Can you work these out from the model? Positions are in its coordinate system, mm. Face numbers are marked on the shaded views. A direction names the side the tool comes from. Give positions to 0.01 mm unless a question says otherwise; leave off trailing zeros. Write each loop counter-clockwise with the first axis right and the second up, starting at its lowest first coordinate (ties: lowest second). Pieces come first, ordered by that corner, then holes. Notation, with made-up numbers: (61, 8) -> (93, 8) arc R29 ccw to (93, 38) -> close; hole circle Ø4 at (16.5, 6.5). An arc over 180 degrees is marked (long way). One line per item, written item: value.
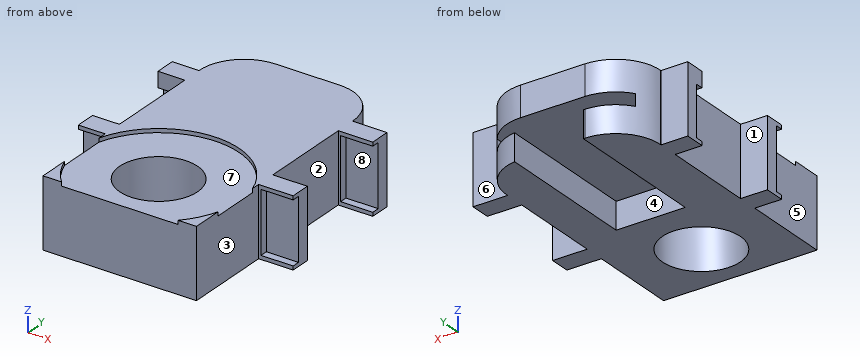
from build123d import *

# Parameters (mm, degrees)
SKETCH2_W           = 20
SKETCH2_H           = 35
BOSS_EXTRUDE1_DEPTH = 9
SKETCH3_W           = 9
SKETCH3_H           = 2.65
BOSS_EXTRUDE2_DEPTH = 14
SKETCH3_2_W         = 9
SKETCH3_2_H         = 2.65
BOSS_EXTRUDE3_DEPTH = 14
SKETCH4_R           = 5.075
CUT_EXTRUDE1_DEPTH  = 10
SKETCH5_R           = 10.5
CUT_EXTRUDE2_DEPTH  = 0.5
SKETCH7_W           = 18
SKETCH7_H           = 1.55
CUT_EXTRUDE3_DEPTH  = 22.2
SKETCH8_W           = 9
SKETCH8_H           = 3.5
CUT_EXTRUDE4_DEPTH  = 19
CUT_EXTRUDE5_DEPTH  = 1
SKETCH10_W          = 3.2
SKETCH10_H          = 6.5
SKETCH10_W_2        = 4.2
SKETCH10_H_2        = 8
CUT_EXTRUDE6_DEPTH  = 1
CUT_EXTRUDE7_DEPTH  = 10


with BuildPart() as part:
    # Sketch2 → Boss-Extrude1 (new body)
    with BuildSketch(Plane.XY):
        with Locations((-6.829268293, 8.069105691)):
            Rectangle(SKETCH2_W, SKETCH2_H)
    extrude(amount=BOSS_EXTRUDE1_DEPTH)

    # Sketch3 → Boss-Extrude2 (add)
    with BuildSketch(Plane(origin=(-6.329268293, 0, 0), x_dir=(0, 0, -1), z_dir=(1, 0, 0))):
        with Locations((-4.5, 18.344105691)):
            Rectangle(SKETCH3_W, SKETCH3_H)
        with Locations((-4.5, 3.494105691)):
            Rectangle(SKETCH3_W, SKETCH3_H)
    extrude(amount=BOSS_EXTRUDE2_DEPTH)

    # Sketch3_2 → Boss-Extrude3 (add)
    with BuildSketch(Plane(origin=(-6.329268293, 0, 0), x_dir=(0, 0, -1), z_dir=(1, 0, 0))):
        with Locations((-4.5, 18.344105691)):
            Rectangle(SKETCH3_2_W, SKETCH3_2_H)
        with Locations((-4.5, 3.494105691)):
            Rectangle(SKETCH3_2_W, SKETCH3_2_H)
    extrude(amount=-BOSS_EXTRUDE3_DEPTH)

    # Sketch4 → Cut-Extrude1 (cut, through all)
    with BuildSketch(Plane.XY.offset(9)):
        with Locations((-6.829268293, -2.173702028)):
            Circle(SKETCH4_R)
    extrude(amount=-CUT_EXTRUDE1_DEPTH, mode=Mode.SUBTRACT)

    # Sketch5 → Cut-Extrude2 (cut)
    with BuildSketch(Plane.XY.offset(9)):
        with Locations((-6.829268293, -2.173702028)):
            Circle(SKETCH5_R)
    extrude(amount=-CUT_EXTRUDE2_DEPTH, mode=Mode.SUBTRACT)

    # Sketch7 → Cut-Extrude3 (cut)
    with BuildSketch(Plane(origin=(0, 25.569105691, 0), x_dir=(1, 0, 0), z_dir=(0, 1, 0))):
        with Locations((-6.829268293, -4.275)):
            Rectangle(SKETCH7_W, SKETCH7_H)
    extrude(amount=-CUT_EXTRUDE3_DEPTH, mode=Mode.SUBTRACT)

    # Sketch8 → Cut-Extrude4 (cut)
    with BuildSketch(Plane(origin=(0, 25.569105691, 0), x_dir=(1, 0, 0), z_dir=(0, 1, 0))):
        with Locations((-6.329268293, -1.75)):
            Rectangle(SKETCH8_W, SKETCH8_H)
    extrude(amount=-CUT_EXTRUDE4_DEPTH, mode=Mode.SUBTRACT)

    # Sketch9 → Cut-Extrude5 (cut)
    with BuildSketch(Plane.XZ.offset(-2.169105691)):
        Polygon((-20.329268293, 8.5), (-17.129268293, 8.5), (-17.129268293, 3.5), (-17.129268293, 1.5), (-17.129268293, 0.5), (-20.329268293, 0.5), (-20.329268293, 1.5), (-20.329268293, 3.5), align=None)
        Polygon((3.470731707, 8.5), (7.670731707, 8.5), (7.670731707, 3.5), (7.670731707, 1.5), (7.670731707, 0.5), (3.470731707, 0.5), (3.470731707, 1.5), (3.470731707, 7.5), align=None)
    extrude(amount=-CUT_EXTRUDE5_DEPTH, mode=Mode.SUBTRACT)

    # Sketch10 → Cut-Extrude6 (cut)
    with BuildSketch(Plane.XZ.offset(-17.019105691)):
        with Locations((-18.729268293, 3.75)):
            Rectangle(SKETCH10_W, SKETCH10_H)
        with Locations((5.570731707, 4.5)):
            Rectangle(SKETCH10_W_2, SKETCH10_H_2)
    extrude(amount=-CUT_EXTRUDE6_DEPTH, mode=Mode.SUBTRACT)

    # Sketch13 → Cut-Extrude7 (cut)
    with BuildSketch(Plane.XY.offset(9)):
        with BuildLine():
            Line((3.170731707, 25.569105691), (-2.629268293, 25.569105691))
            ThreePointArc((-2.629268293, 25.569105691), (1.471951038, 23.870325022), (3.170731707, 19.769105691))
            Line((3.170731707, 19.769105691), (3.170731707, 25.569105691))
        make_face()
        with BuildLine():
            ThreePointArc((-16.829268293, 19.769105691), (-15.130487624, 23.870325022), (-11.029268293, 25.569105691))
            Line((-11.029268293, 25.569105691), (-16.829268293, 25.569105691))
            Line((-16.829268293, 25.569105691), (-16.829268293, 19.769105691))
        make_face()
    extrude(amount=-CUT_EXTRUDE7_DEPTH, mode=Mode.SUBTRACT)


solid = part.part
1) If we section it at D-D (y = -4): Write out the boundary of the cut face in (x, z), and give its area (3 significant figures).
Answer list:
outline: (-16.83, 0) -> (-11.56, 0) -> (-11.56, 8.5) -> (-16.83, 8.5) -> close; (-2.09, 0) -> (3.17, 0) -> (3.17, 8.5) -> (-2.09, 8.5) -> close
area: 89.5 mm^2
2) We'd pull the mould along Y, two halves only. Please class the marked faces 1, 2, 3 and 4: released by +Y, released by -Y, zero draft, split by the parting line, or undercut.
Answer list:
face 1: undercut
face 2: undercut
face 3: zero draft
face 4: released by +Y
3) I need wall thicknesses on L1, parallel to X at y = 12, z = 0.75; L2, parallel to Z at x = -1.5, y = 12; L3, parallel to Y at x = 4.75, z = 5.75. Which ranges of each line are inside material? Lowest first, please.
Answer list:
L1: x = -16.83 to -10.83, -1.83 to 3.17
L2: z = 0 to 3.5, 5.05 to 9
L3: y = 3.17 to 4.82, 18.02 to 19.67
4) If we section it at A-A (x = -9.25): Write out the boundary of the cut face in (y, z).
Answer list:
outline: (-9.43, 0) -> (-6.63, 0) -> (-6.63, 8.5) -> (-9.43, 8.5) -> close; (2.29, 0) -> (6.57, 0) -> (6.57, 3.5) -> (3.37, 3.5) -> (3.37, 5.05) -> (25.57, 5.05) -> (25.57, 9) -> (8.04, 9) -> (8.04, 8.5) -> (2.29, 8.5) -> close
5) Will these pins go through, and if not, where does the flat tip stop? pin 1 (4 mm diameter, centred on x = -18, z = 3, fed in from +Y); pin 2 (1 mm diameter, centred on y = 7, z = 2.5, fed in from +X); pin 3 (5 mm diameter, centred on y = -2, z = 3.5, fed in from -X); pin 4 (1.1 mm diameter, centred on x = -18, y = 17.5, fed in from -Z).
Answer list:
pin 1: stops at y = 22.76
pin 2: stops at x = 3.17
pin 3: stops at x = -16.83
pin 4: stops at z = 0
6) If we section it at B-B (y = 18.5): Write out the boundary of the cut face in (x, z).
Answer list:
outline: (-20.33, 0) -> (-10.83, 0) -> (-10.83, 3.5) -> (-15.83, 3.5) -> (-15.83, 5.05) -> (2.17, 5.05) -> (2.17, 3.5) -> (-1.83, 3.5) -> (-1.83, 0) -> (7.67, 0) -> (7.67, 9) -> (-20.33, 9) -> close
7) For the marked faces 5, 6, 7 and 8, which set-ups out of +Z, -Z, +X, -X, +Y, -Y let a thin tool reach every point of the face, with its end or its side?
Answer list:
face 5: +Z, -Z, -X, -Y
face 6: +Z, -Z, +X, +Y
face 7: +Z
face 8: +X
